Autodesk Inventor part; units mm, degrees
ref_plane "YZ Plane" through (0, 0, 0) normal (1, 0, 0) x (0, 1, 0)
ref_plane "XZ Plane" through (0, 0, 0) normal (0, 1, 0) x (-1, 0, 0)
ref_plane "XY Plane" through (0, 0, 0) normal (0, 0, 1) x (1, 0, 0)
sketch "スケッチ1" plane through (0, 0, 0) normal (0, 0, 1) x (1, 0, 0)
  line L0 (0, 0) -> (0, -20) construction
  line L1 (0, -20) -> (-37.9074, -2.6507) construction
  line L2 (-37.9074, -2.6507) -> (0, 0) construction
  arc A0 (-41.6469, -1.2309) -> (-36.19, -6.2633) centre (-37.9074, -2.6507) ccw
  arc A1 (5.4905, 0.3235) -> (-1.2529, 5.3554) centre (0, 0) ccw
  arc A2 (-6.5, -23) -> (6.5, -23) centre (0, -23) ccw
  arc A3 (3.5, -17) -> (-3.5, -17) centre (0, -17) ccw
  arc A4 (-3.5, -23) -> (3.5, -23) centre (0, -23) ccw
  line L3 (-3.5, -17) -> (-3.5, -23)
  line L4 (3.5, -17) -> (3.5, -23)
  line L5 (0, -23) -> (0, -17) construction
  line L6 (5.4905, 0.3235) -> (6.4887, -16.6176)
  line L7 (6.5, -17) -> (6.5, -23)
  arc A5 (6.5, -17) -> (6.4887, -16.6176) centre (0, -17) ccw
  line L8 (-6.5, -23) -> (-6.5, -17)
  arc A6 (-1.2529, 5.3554) -> (-5.4905, 0.3235) centre (0, 0) ccw construction
  line L9 (-5.4905, 0.3235) -> (-5.7734, -4.4787) construction
  arc A7 (-6.4887, -16.6176) -> (-6.5, -17) centre (0, -17) ccw
  line L10 (-5.8372, -5.5609) -> (-6.4887, -16.6176)
  arc A8 (-5.8372, -5.5609) -> (-7.8781, -3.4437) centre (-7.8338, -5.4432) ccw
  line L11 (-40.6241, 1.4629) -> (-41.6469, -1.2309)
  arc A9 (-26, -3.8454) -> (-36.19, -6.2633) centre (-25.4454, -28.8643) ccw
  line L12 (-26, -3.8454) -> (-7.8781, -3.4437)
  arc A10 (-39.0031, 2.49) -> (-40.6241, 1.4629) centre (-39.1283, 0.8949) ccw
  arc A11 (-39.0031, 2.49) -> (-1.2529, 5.3554) centre (-29.3534, 125.4645) ccw
  line L13 (-26.133, 2.1531) -> (-8.011, 2.5548) construction
  line L14 (-39.1283, 0.8949) -> (-37.9074, -2.6507) construction
  dimension "d0" = 20
  dimension "d2" = 38
  dimension "d3" = 4
  dimension "d13" = 6
  dimension "d14" = 3.5
  dimension "d15" = 6.5
  dimension "d21" = 86
  dimension "d27" = 2
  dimension "d32" = 5.5
  dimension "d35" = 88.73
  dimension "d36" = 3.2683
  dimension "d39" = 1.6
  dimension "d40" = 26
  dimension "d41" = 6
  dimension "d42" = 105
  dimension "d43" = 3.75
extrude "押し出し1" add sketch "スケッチ1" along normal blind 3
hole "穴1" at (-37.9074, -2.6507, 0) at (0, 0, 0) direction (0, 0, 1) diameter 3 end through all
sketch "スケッチ2" plane through (0, 0, 3) normal (0, 0, 1) x (1, 0, 0)
  arc A0 (3.5, -17) -> (-3.5, -17) centre (0, -17) ccw
  line L0 (3.5, -17) -> (3.5, -23)
  arc A1 (-3.5, -23) -> (3.5, -23) centre (0, -23) ccw
  line L1 (-3.5, -23) -> (-3.5, -17)
  point P0 (0, 0)
extrude "押し出し2" add sketch "スケッチ2" against normal blind 0.4
properties part number "COXA_YAW_SUPPORT-LINK_BACK"
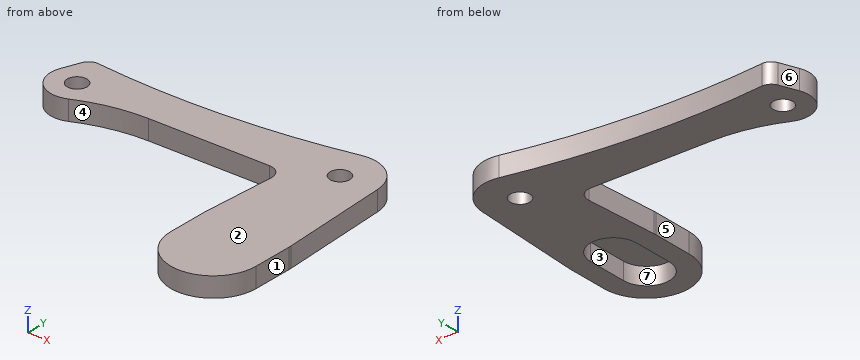
The model under review builds one solid part; all positions refer to its coordinate system, in mm. Face numbers are marked on the shaded views. A direction names the side the tool comes from. Coordinates: 2 decimals unless noted, no trailing zeros. Loops run counter-clockwise (first coordinate to the right, second up) from the corner with the lowest first, then second, coordinate; pieces in that order, holes last.
(1) Consider section D-D, the plane x = -23. Give the boundary of the cut face in (y, z).
Determined:
outline: (-3.78, 0) - (2.28, 0) - (2.28, 3) - (-3.78, 3) - close
(2) Consider section B-B, the plane z = 0.55. Give the boundary of the cut face in (x, y).
Determined:
outline: (-41.65, -1.23) arc R4 ccw to (-36.19, -6.26) arc R25.02 cw to (-26, -3.85) - (-7.88, -3.44) arc R2 cw to (-5.84, -5.56) - (-6.49, -16.62) arc R6.55 ccw to (-6.5, -17) - (-6.5, -23) arc R6.5 ccw to (6.5, -23) - (6.5, -17) arc R6.45 ccw to (6.49, -16.62) - (5.49, 0.32) arc R5.5 ccw to (-1.25, 5.36) arc R123.35 cw to (-39, 2.49) arc R1.6 ccw to (-40.62, 1.46) - close; hole circle Ø3 at (-37.91, -2.65); hole (-3.5, -23) arc R3.5 ccw to (3.5, -23) - (3.5, -17) arc R3.5 ccw to (-3.5, -17) - close; hole circle Ø3 at (0, 0)
(3) Insertion check: P1, Ø1.5, axis at y = -19, z = 1, coming from the -X side; P2, Ø2.5, axis at x = -37.91, y = -2.65, coming from the +Z side. Each pin has a flat end and moves straight along its axis. Give the tip position at first contact, or say it passes through.
Determined:
P1: stops at x = -6.5
P2: passes through
(4) Consider section C-C, the plane y = -10. Give the boundary of the cut face in (x, z), plus the area to 3 significant figures.
Determined:
outline: (-6.1, 0) - (6.1, 0) - (6.1, 3) - (-6.1, 3) - close
area: 36.6 mm2
(5) Tool access review of the marked faces 4, 5, 6 and 7: name each direction out of +Z, -Z, +X, -X, +Y, -Y from which nothing blocks a thin tool from reaching the whole face with its end or side.
Determined:
face 4: +Z, -Z, -Y
face 5: +Z, -Z, -X, -Y
face 6: +Z, -Z, -X, +Y
face 7: -Z
(6) Wall thickness on L1, parallel to Y at x = 0, z = 1.4; L2, parallel to Y at x = 0.5, z = 2.45; L3, parallel to Y at x = 3, z = 0.9: over which ranges is each line inside the solid? List them lowest first.
Determined:
L1: y = -29.5 to -26.5, -13.5 to -1.5, 1.5 to 5.5
L2: y = -29.48 to -26.46, -13.54 to -1.41, 1.41 to 5.48
L3: y = -28.77 to -24.8, -15.2 to 4.61
(7) Consider section A-A, the plane x = 0. Give the boundary of the cut face in (y, z), plus the area to 3 significant figures.
Determined:
outline: (-29.5, 0) - (-26.5, 0) - (-26.5, 2.6) - (-13.5, 2.6) - (-13.5, 0) - (-1.5, 0) - (-1.5, 3) - (-29.5, 3) - close; (1.5, 0) - (5.5, 0) - (5.5, 3) - (1.5, 3) - close
area: 62.2 mm2
(8) Draft analysis for pull direction X (two halves, no side actions). For the marked faces 1, 2 and 3, state which applies: +X half, -X half, draft (parallel to the pull), parting line (faces both ways), or undercut.
Determined:
face 1: +X half
face 2: draft
face 3: undercut
